Can you work these out from the model? Positions are in its coordinate system, mm. Give positions to 0.01 mm unless a question says otherwise; leave off trailing zeros. Order: outer loops, then holes, each group sorted by start corner. A loop starts at its lowest first (then second) coordinate and runs counter-clockwise, first axis right, second up. Notation, with made-up numbers: (-7.5, -36.5) -> (-1.5, -36.5) arc R20 ccw to (-1.5, -0.5) -> close; hole circle Ø5 at (19.5, -11.75). An arc over 180 degrees is marked (long way). Answer as a JSON object with one key per item and string values.
```python
from build123d import *

# Parameters (mm, degrees)
SKETCH2_W            = 300
SKETCH2_H            = 90
BOSS_EXTRUDE1_DEPTH  = 3.175
SKETCH4_W            = 170
SKETCH4_H            = 55
SKETCH4_W_2          = 110
SKETCH4_H_2          = 75
SKETCH4_H_3          = 14
CUT_EXTRUDE2_DEPTH   = 157.636779286
M3_CLEARANCE_HOLE1_D = 3.2
FILLET1_R            = 3
FILLET2_R            = 1


with BuildPart() as part:
    # Sketch2 → Boss-Extrude1 (new body)
    with BuildSketch(Plane(origin=(0, 0, 0), x_dir=(0, 0, -1), z_dir=(1, 0, 0))):
        Rectangle(SKETCH2_W, SKETCH2_H)
    extrude(amount=BOSS_EXTRUDE1_DEPTH)

    # Sketch4 → Cut-Extrude2 (cut, through all)
    with BuildSketch(Plane(origin=(3.175, 0, 0), x_dir=(0, 0, -1), z_dir=(1, 0, 0))):
        with Locations((-57, -12.5)):
            Rectangle(SKETCH4_W, SKETCH4_H)
        with Locations((90.2375, -2.7375)):
            Rectangle(SKETCH4_W_2, SKETCH4_H_2)
        with Locations((-57, 30)):
            Rectangle(SKETCH4_W, SKETCH4_H_3)
    extrude(amount=-CUT_EXTRUDE2_DEPTH, mode=Mode.SUBTRACT)

    # M3 Clearance Hole1 (through all)
    with Locations(Plane(origin=(3.175, 0, 0), x_dir=(0, 0, -1), z_dir=(1, 0, 0))):
        with Locations((-137.5, 42.61875), (0, 42.61875), (137.5, 42.61875), (137.5, -42.61875), (0, -42.61875), (-137.5, -42.61875)):
            Hole(M3_CLEARANCE_HOLE1_D / 2)

    # Fillet1
    fillet1_edges = [part.edges().sort_by_distance(p)[0] for p in [
        (1.5875, 34.7625, -145.2375),
        (1.5875, -40.2375, -145.2375),
        (1.5875, -40.2375, -35.2375),
        (1.5875, 34.7625, -35.2375),
        (1.5875, -40, 142),
        (1.5875, 15, 142),
        (1.5875, 15, -28),
        (1.5875, -40, -28),
        (1.5875, 23, 142),
        (1.5875, 37, 142),
        (1.5875, 37, -28),
        (1.5875, 23, -28),
    ]]
    fillet(fillet1_edges, radius=FILLET1_R)

    # Fillet2
    fillet2_edges = [part.edges().sort_by_distance(p)[0] for p in [
        (1.5875, -45, -150),
        (1.5875, -45, 150),
        (1.5875, 45, 150),
        (1.5875, 45, -150),
    ]]
    fillet(fillet2_edges, radius=FILLET2_R)


solid = part.part
```
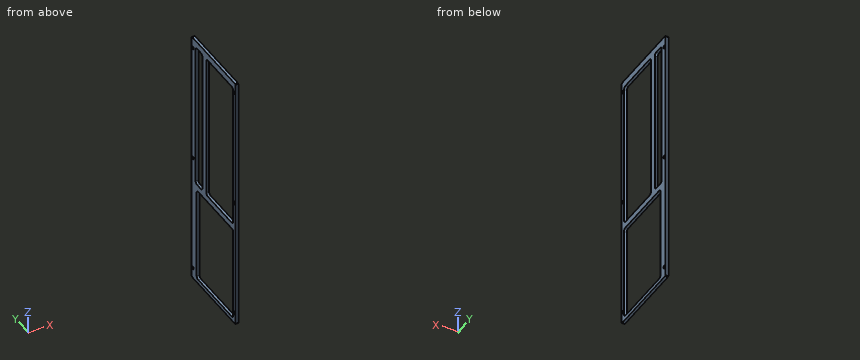
1. If we section it at D-D on x = 2.05: Count the separate pieces of the cut face and the enclosed holes in it, then the cut area to 3 significant figures.
Worked answers:
{"separate pieces": "1", "enclosed holes": "9", "area": "6,990 mm²"}
2. If we section it at A-A on z = 112: Please give me the cut outline in (x, y) (3 decimals).
Worked answers:
{"outline": "(0, -45) -> (3.175, -45) -> (3.175, -40) -> (0, -40) -> close; (0, 15) -> (3.175, 15) -> (3.175, 23) -> (0, 23) -> close; (0, 37) -> (3.175, 37) -> (3.175, 45) -> (0, 45) -> close"}
3. Please list where these lines run through material, in increasing order: L1, parallel to Z at x = 2, y = 26; L2, parallel to Y at x = 3, z = 0; L3, parallel to Y at x = 0.5, z = 89.
Worked answers:
{"L1": "-150 to -145.24, -35.24 to -28, 142 to 150", "L2": "-45 to -44.22, -41.02 to -40, 15 to 23, 37 to 41.02, 44.22 to 45", "L3": "-45 to -40, 15 to 23, 37 to 45"}
4. If we section it at C-C on z = -62: Please give me the cut outline in (x, y) (1 decimal), then the cut area to 3 significant figures.
Worked answers:
{"outline": "(0, -45) -> (3.2, -45) -> (3.2, -40.2) -> (0, -40.2) -> close; (0, 34.8) -> (3.2, 34.8) -> (3.2, 45) -> (0, 45) -> close", "area": "47.6 mm²"}
5. If we section it at B-B on y = -30: Please give me the cut outline in (x, z) (1 decimal), then the cut area to 3 significant figures.
Worked answers:
{"outline": "(0, -150) -> (3.2, -150) -> (3.2, -145.2) -> (0, -145.2) -> close; (0, -35.2) -> (3.2, -35.2) -> (3.2, -28) -> (0, -28) -> close; (0, 142) -> (3.2, 142) -> (3.2, 150) -> (0, 150) -> close", "area": "63.5 mm²"}
